from build123d import *

# Parameters (mm, degrees)
BOSS_EXTRUDE1_DEPTH = 8
CUT_EXTRUDE2_DEPTH  = 3
SKETCH3_R           = 4
CUT_EXTRUDE1_DEPTH  = 235.746671968
BOSS_EXTRUDE2_DEPTH = 8


with BuildPart() as part:
    # Sweep1: sweep along a path in Sketch2
    with BuildLine(Plane(origin=(0, 0, 0), x_dir=(0, 0, -1), z_dir=(1, 0, 0))) as sweep1_path:
        Line((150, 92), (-150, 92))
        ThreePointArc((-150, 92), (-165.556349186, 85.556349186), (-172, 70))
        Line((-172, 70), (-172, -70))
        ThreePointArc((-172, -70), (-165.556349186, -85.556349186), (-150, -92))
        Line((-150, -92), (150, -92))
        ThreePointArc((150, -92), (165.556349186, -85.556349186), (172, -70))
        Line((172, -70), (172, 70))
        ThreePointArc((172, 70), (165.556349186, 85.556349186), (150, 92))
    # Sketch1 → Sweep1 (sweep)
    with BuildSketch(Plane.XY):
        Polygon((-3, 121), (-3, 81), (-6, 81), (-6, 71), (-11, 71), (-11, 121), align=None)
    sweep(path=sweep1_path.line)

    # Sketch5 → Boss-Extrude1 (add)
    with BuildSketch(Plane.ZY.offset(11)):
        with BuildLine():
            Line((201, -70), (201, 70))
            ThreePointArc((201, 70), (186.062445841, 106.062445841), (150, 121))
            Line((150, 121), (-150, 121))
            ThreePointArc((-150, 121), (-186.062445841, 106.062445841), (-201, 70))
            Line((-201, 70), (-201, -70))
            ThreePointArc((-201, -70), (-186.062445841, -106.062445841), (-150, -121))
            Line((-150, -121), (150, -121))
            ThreePointArc((150, -121), (186.062445841, -106.062445841), (201, -70))
        make_face()
        with BuildLine():
            Line((0, 71), (-150, 71))
            ThreePointArc((-150, 71), (-150.707106781, 70.707106781), (-151, 70))
            Line((-151, 70), (-151, -70))
            ThreePointArc((-151, -70), (-150.707106781, -70.707106781), (-150, -71))
            Line((-150, -71), (150, -71))
            ThreePointArc((150, -71), (150.707106781, -70.707106781), (151, -70))
            Line((151, -70), (151, 70))
            ThreePointArc((151, 70), (150.707106781, 70.707106781), (150, 71))
            Line((150, 71), (0, 71))
        make_face(mode=Mode.SUBTRACT)
    extrude(amount=-BOSS_EXTRUDE1_DEPTH)

    # Sketch7 → Cut-Extrude2 (cut)
    with BuildSketch(Plane(origin=(-3, 0, 0), x_dir=(0, 0, -1), z_dir=(1, 0, 0))):
        with BuildLine():
            Line((161, -70), (161, 70))
            ThreePointArc((161, 70), (157.778174593, 77.778174593), (150, 81))
            Line((150, 81), (-150, 81))
            ThreePointArc((-150, 81), (-157.778174593, 77.778174593), (-161, 70))
            Line((-161, 70), (-161, -70))
            ThreePointArc((-161, -70), (-157.778174593, -77.778174593), (-150, -81))
            Line((-150, -81), (150, -81))
            ThreePointArc((150, -81), (157.778174593, -77.778174593), (161, -70))
        make_face()
    extrude(amount=-CUT_EXTRUDE2_DEPTH, mode=Mode.SUBTRACT)

    # Sketch3 → Cut-Extrude1 (cut, through all)
    with BuildSketch(Plane(origin=(-3, 0, 0), x_dir=(0, 0, -1), z_dir=(1, 0, 0))):
        with Locations((-188.5, 0)):
            Circle(SKETCH3_R)
        with Locations(Location((188.5, 0, 0), (0, 0, 180))):
            Circle(SKETCH3_R)
    extrude(amount=-CUT_EXTRUDE1_DEPTH, mode=Mode.SUBTRACT)

    # Sketch8 → Boss-Extrude2 (add)
    with BuildSketch(Plane(origin=(-3, 0, 0), x_dir=(0, 0, -1), z_dir=(1, 0, 0))):
        with BuildLine():
            Line((-201, -70), (-201, 70))
            ThreePointArc((-201, 70), (-203.099371321, 63.066247547), (-208.692307692, 58.461538462))
            ThreePointArc((-208.692307692, 58.461538462), (-217.641005887, 51.094003925), (-221, 40))
            Line((-221, 40), (-221, -40))
            ThreePointArc((-221, -40), (-217.641005887, -51.094003925), (-208.692307692, -58.461538462))
            ThreePointArc((-208.692307692, -58.461538462), (-203.099371321, -63.066247547), (-201, -70))
        make_face()
    boss_extrude2 = extrude(amount=-BOSS_EXTRUDE2_DEPTH)

    # Mirror1: Boss-Extrude2 across plane
    add(boss_extrude2.mirror(Plane.XY))


solid = part.part
The listing builds one solid part. Answer for the finished solid, in the listing's coordinates (mm). A direction names the side the tool comes from. Give positions to 0.01 mm unless a question says otherwise; leave off trailing zeros. Write each loop counter-clockwise with the first axis right and the second up, starting at its lowest first coordinate (ties: lowest second). Pieces come first, ordered by that corner, then holes. Notation, with made-up numbers: (20.5, 36.5) -> (27.5, 36.5) arc R31 ccw to (27.5, 69.5) -> close; hole circle Ø2 at (-35.75, 4). An arc over 180 degrees is marked (long way). Use a Markdown table: item, result.
(1) Section A-A, the plane z = 122.5 is taken. Determine the outline of the cut face in (x, y).
Return value:
| item | result |
|---|---|
| outline | (-11, -121) -> (-3, -121) -> (-3, -81) -> (-6, -81) -> (-6, -71) -> (-11, -71) -> close; (-11, 71) -> (-6, 71) -> (-6, 81) -> (-3, 81) -> (-3, 121) -> (-11, 121) -> close |
(2) Flat-ended cylindrical pins translate along their axes: P1, Ø4, axis at x = -7, y = -75, coming from the +Z side; P2, Ø6.5, axis at y = 0, z = 188.5, coming from the -X side; P3, Ø3, axis at x = -5, y = 56, coming from the +Z side (3 decimals). Find the tip coordinate at first contact, or state that the pin passes through.
Return value:
| item | result |
|---|---|
| P1 | z = 200.91 |
| P2 | through |
| P3 | z = 214.775 |
(3) For faces 1 (the flat face through (-7, -121, -2)), 2 (the cylindrical face through (-4.479, -77.863, -157.692)), determine the directions among +Z, -Z, +X, -X, +Y, -Y from which every point of the face is accessible in a straight line to the end or side of a thin tool.
Return value:
| item | result |
|---|---|
| face 1 | +Z, -Z, +X, -X, -Y |
| face 2 | +X |
(4) Section C-C, the plane y = -51.5 is taken. Determine the outline of the cut face in (x, z), then the cut area to 3 significant figures.
Return value:
| item | result |
|---|---|
| outline | (-11, -217.36) -> (-3, -217.36) -> (-3, -161) -> (-6, -161) -> (-6, -151) -> (-11, -151) -> close; (-11, 151) -> (-6, 151) -> (-6, 161) -> (-3, 161) -> (-3, 217.36) -> (-11, 217.36) -> close |
| area | 1,000 mm2 |
(5) Determine the mould class of faces 3 (the cylindrical face through (-6.94, 51.23, -217.55)), 4 (the cylindrical face through (-6.94, -50.96, -217.73)), 5 (the flat face through (-6, -72, 13)) for opening direction Y: released by +Y, released by -Y, zero draft, split by the parting line, or undercut.
Return value:
| item | result |
|---|---|
| face 3 | released by +Y |
| face 4 | released by -Y |
| face 5 | undercut |
(6) Section B-B, the plane x = -8.5 is taken. Determine the outline of the cut face in (y, z).
Return value:
| item | result |
|---|---|
| outline | (-121, -150) arc R51 ccw to (-70, -201) arc R12.5 cw to (-58.46, -208.69) arc R20 ccw to (-40, -221) -> (40, -221) arc R20 ccw to (58.46, -208.69) arc R12.5 cw to (70, -201) arc R51 ccw to (121, -150) -> (121, 150) arc R51 ccw to (70, 201) arc R12.5 cw to (58.46, 208.69) arc R20 ccw to (40, 221) -> (-40, 221) arc R20 ccw to (-58.46, 208.69) arc R12.5 cw to (-70, 201) arc R51 ccw to (-121, 150) -> close; hole (-71, -150) arc R1 ccw to (-70, -151) -> (70, -151) arc R1 ccw to (71, -150) -> (71, 150) arc R1 ccw to (70, 151) -> (-70, 151) arc R1 ccw to (-71, 150) -> close; hole circle Ø8 at (0, -188.5); hole circle Ø8 at (0, 188.5) |
(7) Find the intervals of material crossed by probe 1 along Y at (x, z) = (-6.25, 127.5); probe 2 along Z at (x, y) = (-4.5, 15); probe 3 along Z at (x, y) = (-9.5, -37), in increasing order. Write a range as from..to.
Return value:
| item | result |
|---|---|
| probe 1 | -121..-71, 71..121 |
| probe 2 | -221..-161, 161..221 |
| probe 3 | -221..-151, 151..221 |
(8) Section D-D, the plane y = 104.5 is taken. Determine the outline of the cut face in (x, z).
Return value:
| item | result |
|---|---|
| outline | (-11, -187.56) -> (-3, -187.56) -> (-3, 187.56) -> (-11, 187.56) -> close |
